Check sheet for the modelled part. Datum: model origin and axes. Units: mm. A direction names the side the tool comes from. Give positions to 0.01 mm unless a question says otherwise; leave off trailing zeros. Order: outer loops, then holes, each group sorted by start corner. A loop starts at its lowest first (then second) coordinate and runs counter-clockwise, first axis right, second up.
Autodesk Fusion 360 part; units mm, degrees
sketch "Sketch1" plane through (0, 0, 0) normal (0, 0, 1) x (1, 0, 0)
  circle A0 centre (0, 0) radius 15.5
  circle A1 centre (0, 0) radius 1
  dimension "d1" = 31
  dimension "d2" = 2
extrude "Extrude1" add sketch "Sketch1" along normal blind 3
sketch "Sketch2" plane through (0, 0, 3) normal (0, 0, 1) x (-1, 0, 0)
  circle A0 centre (0, 0) radius 1
  circle A1 centre (0, 0) radius 15.5
  circle A2 centre (12, 0) radius 3
  circle A3 centre (-12, 0) radius 3
  line L0 (15.5, 0) -> (12, 0)
  line L1 (-12, 0) -> (-15.5, 0)
  dimension "d7" = 6
extrude "Extrude2" add sketch "Sketch2" along normal blind 50 contours A3 | A2
1) Section check D-D, the plane x = 12. Record the cut outline in (y, z), then the cut area to 3 significant figures.
Recorded:
outline: (-9.81, 0) - (9.81, 0) - (9.81, 3) - (3, 3) - (3, 53) - (-3, 53) - (-3, 3) - (-9.81, 3) - close
area: 359 mm2
2) Section check C-C, the plane z = 39.5. Record the cut outline in (x, y), then the cut area to 3 significant figures.
Recorded:
outline: circle Ø6 at (-12, 0); circle Ø6 at (12, 0)
area: 56.5 mm2
3) Material ranges on L1, parallel to Y at x = 0, z = 1.6; L2, parallel to Z at x = 7.5, y = 11.5; L3, parallel to Y at x = 13, z = 45.5, recorded low to high.
Recorded:
L1: y = -15.5 to -1, 1 to 15.5
L2: z = 0 to 3
L3: y = -2.83 to 2.83
4) Draft check along X on faces 1 (the face through (-12, 0, 53)), 2 (the face through (14.4, -1.8, 27.6)), 3 (the face through (-2.018, -15.368, 1.479)). Enter one of: +X half, -X half, draft (parallel to the pull), parting line (faces both ways), or undercut.
Recorded:
face 1: draft
face 2: undercut
face 3: parting line
5) Set-up check for faces 4 (the face through (-9.6, -1.8, 27.6)), 5 (the face through (0, -3, 0)): record each of +Z, -Z, +X, -X, +Y, -Y from which the full face is reachable in a straight line by a thin tool's end or side.
Recorded:
face 4: +Z
face 5: -Z, +X, -X, +Y, -Y
6) Section check B-B, the plane x = 0. Record the cut outline in (y, z), then the cut area to 3 significant figures.
Recorded:
outline: (-15.5, 0) - (-1, 0) - (-1, 3) - (-15.5, 3) - close; (1, 0) - (15.5, 0) - (15.5, 3) - (1, 3) - close
area: 87.0 mm2
7) Depth check by flat-ended pin: pin 1 Ø1 at (x, z) = (10, 33) entering from +Y; pin 2 Ø1 at (x, y) = (-3.5, -2) entering from +Z; pin 3 Ø1 at (y, z) = (1.5, 28.5) entering from -X. Enter the tip coordinate at first touch or a pass-through.
Recorded:
pin 1: stops at y = 2.6
pin 2: stops at z = 3
pin 3: stops at x = -14.83
8) Section check A-A, the plane y = 0. Record the cut outline in (x, z).
Recorded:
outline: (-15.5, 0) - (-1, 0) - (-1, 3) - (-9, 3) - (-9, 53) - (-15, 53) - (-15, 3) - (-15.5, 3) - close; (1, 0) - (15.5, 0) - (15.5, 3) - (15, 3) - (15, 53) - (9, 53) - (9, 3) - (1, 3) - close
